```python
from build123d import *

# Parameters (mm, degrees)
CROQUIS1_W              = 25
CROQUIS1_H              = 65
SALIENTE_EXTRUIR1_DEPTH = 15.5
CROQUIS2_R              = 6
CORTAR_EXTRUIR1_DEPTH   = 7
REDONDEO1_R             = 10
REDONDEO2_R             = 5
CROQUIS3_R              = 5
CORTAR_EXTRUIR2_DEPTH   = 5.5
REDONDEO3_R             = 5


with BuildPart() as part:
    # Croquis1 → Saliente-Extruir1 (new, symmetric)
    with BuildSketch(Plane.XY):
        with Locations((10.230951989, -15.239848308)):
            Rectangle(CROQUIS1_W, CROQUIS1_H)
    extrude(amount=SALIENTE_EXTRUIR1_DEPTH, both=True)

    # Croquis2 → Cortar-Extruir1 (cut)
    with BuildSketch(Plane.XY.offset(15.5)):
        with BuildLine():
            Line((-2.269048011, 9.260151692), (-2.269048011, 26.058320898))
            Line((-2.269048011, 26.058320898), (22.730951989, 26.058320898))
            Line((22.730951989, 26.058320898), (22.730951989, 9.260151692))
            Line((22.730951989, 9.260151692), (22.730951989, 3.260151692))
            Line((22.730951989, 3.260151692), (21.196808088, 3.260151692))
            ThreePointArc((21.196808088, 3.260151692), (10.230951989, -3.239848308), (-0.734904111, 3.260151692))
            Line((-0.734904111, 3.260151692), (-2.269048011, 3.260151692))
            Line((-2.269048011, 3.260151692), (-2.269048011, 9.260151692))
        make_face()
        with Locations((10.230951989, 9.260151692)):
            Circle(CROQUIS2_R, mode=Mode.SUBTRACT)
    cortar_extruir1 = extrude(amount=-CORTAR_EXTRUIR1_DEPTH, mode=Mode.SUBTRACT)

    # Simetría1: Cortar-Extruir1 across plane
    add(cortar_extruir1.mirror(Plane.XY), mode=Mode.SUBTRACT)

    # Redondeo1
    redondeo1_edges = [part.edges().sort_by_distance(p)[0] for p in [
        (-2.269048011, 17.260151692, 0),
        (22.730951989, 17.260151692, 0),
    ]]
    fillet(redondeo1_edges, radius=REDONDEO1_R)

    # Redondeo2
    redondeo2_edges = [part.edges().sort_by_distance(p)[0] for p in [
        (22.730951989, -22.239848308, -15.5),
        (22.730951989, -22.239848308, 15.5),
        (-2.269048011, -22.239848308, 15.5),
        (-2.269048011, -22.239848308, -15.5),
    ]]
    fillet(redondeo2_edges, radius=REDONDEO2_R)

    # Croquis3 → Cortar-Extruir2 (cut)
    with BuildSketch(Plane.XZ.offset(47.739848308)):
        with Locations(Location((10.230951989, 0, 0), (0, 0, 270))):
            Circle(CROQUIS3_R)
    extrude(amount=-CORTAR_EXTRUIR2_DEPTH, mode=Mode.SUBTRACT)

    # Redondeo3
    redondeo3_edges = [part.edges().sort_by_distance(p)[0] for p in [
        (22.730951989, -47.739848308, 0),
        (10.230951989, -47.739848308, -15.5),
        (10.230951989, -47.739848308, 15.5),
        (-2.269048011, -47.739848308, 0),
        (-0.804581917, -47.739848308, -14.035533906),
        (-0.804581917, -47.739848308, 14.035533906),
        (21.266485895, -47.739848308, 14.035533906),
        (21.266485895, -47.739848308, -14.035533906),
    ]]
    fillet(redondeo3_edges, radius=REDONDEO3_R)


solid = part.part
```
Could you check a few things on this model? Use its own coordinates, in mm. A direction names the side the tool comes from. Round coordinates to 2 decimals unless told otherwise and drop trailing zeros. Order: outer loops, then holes, each group sorted by start corner. A loop starts at its lowest first (then second) coordinate and runs counter-clockwise, first axis right, second up. Notation, with made-up numbers: (-35.5, -5) -> (17.5, -5) arc R35 cw to (17.5, 31) -> close; hole circle Ø7 at (37, 72.25). An arc over 180 degrees is marked (long way). One line per question, with ' | ' between items.
Q1. If I drill on line 1 (X direction, y = -45.5, z = 0); line 2 (X direction, y = -45.3, z = 0); line 3 (Y direction, x = 9, z = -2), over which ranges is the centre line in solid material (lowest first)? Write a range as from..to.
Computed values:
line 1: -1.44..5.23, 15.23..21.9 | line 2: -1.56..5.23, 15.23..22.03 | line 3: -42.24..17.26
Q2. If we section it at D-D on y = 4: Write out the boundary of the cut face in (x, z).
Computed values:
outline: (-2.27, -8.5) -> (7.34, -8.5) -> (7.34, -15.5) -> (13.12, -15.5) -> (13.12, -8.5) -> (22.73, -8.5) -> (22.73, 8.5) -> (13.12, 8.5) -> (13.12, 15.5) -> (7.34, 15.5) -> (7.34, 8.5) -> (-2.27, 8.5) -> close
Q3. If we section it at B-B on z = 0: Write out the boundary of the cut face in (x, y).
Computed values:
outline: (-2.27, -42.74) arc R5 ccw to (2.73, -47.74) -> (5.23, -47.74) -> (5.23, -42.24) -> (15.23, -42.24) -> (15.23, -47.74) -> (17.73, -47.74) arc R5 ccw to (22.73, -42.74) -> (22.73, 7.26) arc R10 ccw to (12.73, 17.26) -> (7.73, 17.26) arc R10 ccw to (-2.27, 7.26) -> close
Q4. If we section it at C-C on x = 17: Write out the boundary of the cut face in (y, z).
Computed values:
outline: (-47.74, -10.5) arc R5 ccw to (-42.74, -15.5) -> (-1.25, -15.5) -> (-1.25, -8.5) -> (16.3, -8.5) -> (16.3, 8.5) -> (-1.25, 8.5) -> (-1.25, 15.5) -> (-42.74, 15.5) arc R5 ccw to (-47.74, 10.5) -> close
Q5. If we section it at A-A on y = -25: Write out the boundary of the cut face in (x, z).
Computed values:
outline: (-2.27, -10.5) arc R5 ccw to (2.73, -15.5) -> (17.73, -15.5) arc R5 ccw to (22.73, -10.5) -> (22.73, 10.5) arc R5 ccw to (17.73, 15.5) -> (2.73, 15.5) arc R5 ccw to (-2.27, 10.5) -> close
Q6. I'm going to push a flat-ended pin straight in: pin 1 (0.5 mm diameter, centred on x = -2, z = 12, fed in from +Y). Where does the tip first touch, or does it pass through?
Computed values:
pin 1: y = 3.26
Q7. We'd pull the mould along X, two halves only. Please class faces 1 (the face through (-0.84, -19.42, 14)), 2 (the face through (10, 3, -8.5)), 3 (the face through (10, -42.24, 0)), 4 (the face through (22, 3.26, -11)): released by +X, released by -X, zero draft, split by the parting line, or undercut.
Computed values:
face 1: released by -X | face 2: undercut | face 3: undercut | face 4: zero draft
Q8. Which directions (+Z, -Z, +X, -X, +Y, -Y) give clear straight access to the entire face, cutting with the end or side of a thin tool? Please do faces 5 (the face through (10.42, -3.24, -12.05)), 6 (the face through (-1, 3.26, 11)), 7 (the face through (8.93, 3.403, 12.049)).
Computed values:
face 5: -Z | face 6: +Z, -X, +Y | face 7: +Z
